```python
from build123d import *

# Parameters (mm, degrees)
SKETCH_1_R          = 10
EXTRUDE_1_DEPTH     = 45
CUT_EXTRUDE_1_DEPTH = 22.5
SKETCH_4_W          = 29.063503474
SKETCH_4_H          = 6
CUT_EXTRUDE_2_DEPTH = 20
SKETCH_5_R          = 2.25
CUT_EXTRUDE_3_DEPTH = 15
SKETCH_6_R          = 3
CUT_EXTRUDE_4_DEPTH = 23


with BuildPart() as part:
    # 草图1 → 凸台-拉伸1 (new body)
    with BuildSketch(Plane.XY):
        with Locations(Location((0, 0, 0), (0, 0, 180))):
            Circle(SKETCH_1_R)
    extrude(amount=EXTRUDE_1_DEPTH)

    # 草图2 → 切除-拉伸1 (cut, symmetric)
    with BuildSketch(Plane(origin=(0, 0, 0), x_dir=(1, 0, 0), z_dir=(0, 1, 0))):
        with BuildLine():
            Line((3, -45), (3, -25))
            ThreePointArc((3, -25), (0, -22), (-3, -25))
            Line((-3, -25), (-3, -45))
            Line((-3, -45), (3, -45))
        make_face()
    extrude(amount=CUT_EXTRUDE_1_DEPTH, both=True, mode=Mode.SUBTRACT)

    # 草图4 → 切除-拉伸2 (cut)
    with BuildSketch(Plane.XY.offset(45)):
        Rectangle(SKETCH_4_W, SKETCH_4_H)
    extrude(amount=-CUT_EXTRUDE_2_DEPTH, mode=Mode.SUBTRACT)

    # 草图5 → 切除-拉伸3 (cut)
    with BuildSketch(Plane(origin=(0, 0, 0), x_dir=(-1, 0, 0), z_dir=(0, 0, -1))):
        Circle(SKETCH_5_R)
    extrude(amount=-CUT_EXTRUDE_3_DEPTH, mode=Mode.SUBTRACT)

    # 草图6 → 切除-拉伸4 (cut, symmetric)
    with BuildSketch(Plane.ZY):
        with Locations((25, 0)):
            Circle(SKETCH_6_R)
    extrude(amount=CUT_EXTRUDE_4_DEPTH, both=True, mode=Mode.SUBTRACT)


solid = part.part
```
Design review of the part built by this model. Coordinates are the model's own, in mm. A direction names the side the tool comes from. Give positions to 0.01 mm unless a question says otherwise; leave off trailing zeros. Order: outer loops, then holes, each group sorted by start corner. A loop starts at its lowest first (then second) coordinate and runs counter-clockwise, first axis right, second up. Notation, with made-up numbers: (75.25, 48) - (82.25, 48) arc R7 cw to (82.25, 59) - close; hole circle Ø11 at (56.5, -30). An arc over 180 degrees is marked (long way). Use a Markdown table: item, result. Add a question column.
(1) Mouldability with a two-part tool opening along X and no side actions: class faces 4 (the face through (-9.54, -3, 22.18)), 5 (the face through (0, 0, 15)), 6 (the face through (6, 5, 45)) as +X half, -X half, draft (parallel to the pull), parting line (faces both ways), or undercut.
(2) Clearance check with flat-ended pins moving along their axes: P1, Ø2, axis at x = 5, z = 39.5, coming from the -Y side; P2, Ø7, axis at x = 6, z = 34.5, coming from the +Y side; P3, Ø2, axis at y = -7.5, z = 15, coming from the -X side. State where each tip first meets the part, or that it passes through.
(3) Add section D-D on x = -1.25. Give the boundary of the cut face in (y, z), then the cut area to 3 significant figures.
(4) Add section A-A on z = 31.5. Give the boundary of the cut face in (x, y), then the cut area to 3 significant figures.
(5) Add section B-B on z = 10. Give the boundary of the cut face in (x, y).
(6) Machinability: for faces 1 (the face through (0.29, 2.23, 7.4)), 2 (the face through (3, 6, 35)), 3 (the face through (-6, 3, 35)), which of the approach directions +Z, -Z, +X, -X, +Y, -Y give a long, thin tool a straight path to every point of the face, cutting with its end or side? Answer none if there is none.
(7) Add section C-C on y = -1.5. Give the boundary of the cut face in (x, z), then the cut area to 3 significant figures.
(8) Wall thickness on probe 1 along Y at (x, z) = (0, 4.75); probe 2 along Z at (x, y) = (-8.5, 0.25); probe 3 along X at (y, z) = (4.75, 33.5): over which ranges is each line inside the solid? List them lowest first. Write a range as [from, to].
Report:
| question | item | result |
|---|---|---|
| 1 | face 4 | parting line |
| 1 | face 5 | undercut |
| 1 | face 6 | draft |
| 2 | P1 | stops at y = -9.17 |
| 2 | P2 | stops at y = 9.54 |
| 2 | P3 | stops at x = -7.6 |
| 3 | outline | (-9.92, 0) - (-1.87, 0) - (-1.87, 15) - (1.87, 15) - (1.87, 0) - (9.92, 0) - (9.92, 22.27) - (1.25, 22.27) arc R3 cw to (-1.25, 22.27) - (-9.92, 22.27) - close |
| 3 | area | 385 mm² |
| 4 | outline | (-9.54, -3) arc R10 ccw to (-3, -9.54) - (-3, -3) - close; (-9.54, 3) - (-3, 3) - (-3, 9.54) arc R10 ccw to start; (3, -9.54) arc R10 ccw to (9.54, -3) - (3, -3) - close; (3, 3) - (9.54, 3) arc R10 ccw to (3, 9.54) - close |
| 4 | area | 114 mm² |
| 5 | outline | circle Ø20 at (0, 0); hole circle Ø4.5 at (0, 0) |
| 6 | face 1 | -Z |
| 6 | face 2 | +Z, +Y, -Y |
| 6 | face 3 | +Z, +X, -X |
| 7 | outline | (-9.89, 0) - (-1.68, 0) - (-1.68, 15) - (1.68, 15) - (1.68, 0) - (9.89, 0) - (9.89, 22.4) - (1.5, 22.4) arc R3 cw to (-1.5, 22.4) - (-9.89, 22.4) - close |
| 7 | area | 392 mm² |
| 8 | probe 1 | y = [-10, -2.25], [2.25, 10] |
| 8 | probe 2 | z = [0, 22.01] |
| 8 | probe 3 | x = [-8.8, -3], [3, 8.8] |
